from build123d import *

# Parameters (mm, degrees)
F0_R     = 31.75
F0_R_2   = 27.94
F1_DEPTH = 38.1
F2_R     = 31.75
F3_DEPTH = 5.08
F4_R     = 6.35
F5_DEPTH = 61.976


with BuildPart() as f1:
    # F0 (on Front) → F1 (new body)
    with BuildSketch(Plane.XZ):
        Circle(F0_R)
        Circle(F0_R_2, mode=Mode.SUBTRACT)
    extrude(amount=F1_DEPTH)

    # F2 (on Front) → F3 (join)
    with BuildSketch(Plane.XZ):
        with Locations((0.1314867404, -0.3395704844)):
            Circle(F2_R)
    extrude(amount=-F3_DEPTH)

    # F4 (on Top) → F5 (cut, symmetric)
    with BuildSketch(Plane.XY):
        with Locations((0, -20.52645199)):
            Circle(F4_R)
    extrude(amount=F5_DEPTH, both=True, mode=Mode.SUBTRACT)


solid = f1.part
Build history of the part. All positions in model axes, mm. A direction names the side the tool comes from. Round coordinates to 2 decimals unless told otherwise and drop trailing zeros. Write each loop counter-clockwise with the first axis right and the second up, starting at its lowest first coordinate (ties: lowest second). Pieces come first, ordered by that corner, then holes. Notation, with made-up numbers: M -17,-17.75 L -8,-17.75 A22 cw -8,-5.75 Z; hole C 62,-3.75 d3. An arc over 180 degrees is marked long. Answer as a JSON object with one key per item and string values. Group by question number.
(1) Cut at C-C (z = 25.5). Give the cut face in (x, y), and give its area (3 significant figures).
(2) Cut at A-A (x = 0). Give the cut face in (y, z), and give its area (3 significant figures).
(3) Mould opens along Z. For faces 3 (the cylindrical face through (12.89, -18.78, -24.79)), 4 (the cylindrical face through (30.415, 2.504, 9.197)), 5 (the flat face through (-0.1, -38.1, -28.1)) say: pulls with the +Z half, pulls with the -Z half, needs draft (parallel to the pull), parting line crosses it, or undercut.
(4) Flat gauge pins, fed straight in: pin 1 (10 mm diameter, centred on y = -7, z = 1.5, fed in from -X); pin 2 (10 mm diameter, centred on x = 0, y = -20.53, fed in from -Z); pin 3 (8 mm diameter, centred on x = -24, y = -16.5, fed in from +Z); pin 4 (20.5 mm diameter, centred on x = 0, y = -20.53, fed in from -Z). Where does each tip first touch, or does it go through?
(5) Cut at D-D (y = -34). Give the cut face in (x, z).
(6) Drill centre lines: L1, parallel to Y at x = 0, z = -30.2; L2, parallel to X at y = -11, z = 0.5. Where is each one in solid material? Low to high.
(7) Cut at B-B (y = -19). Give the cut face in (x, z).
(8) Which spindle directions (+Z, -Z, +X, -X, +Y, -Y) get a long thin tool onto all of the face, cutting with end or side? Do faces 1 (the cylindrical face through (-6.883, -18.783, -30.995)), 2 (the flat face through (0, 5.08, 0)). Say none if no direction does.
Responses:
{
 "1": {"outline": "M -18.92,-38.1 L -11.42,-38.1 L -11.42,0 L 11.42,0 L 11.42,-38.1 L 18.92,-38.1 L 18.92,0 L 18.58,0 L 18.58,5.08 L -18.32,5.08 L -18.32,0 L -18.92,0 Z", "area": "759 mm2"},
 "2": {"outline": "M -38.1,-31.75 L -26.88,-31.75 L -26.88,-27.94 L -38.1,-27.94 Z; M -38.1,27.94 L -26.88,27.94 L -26.88,31.75 L -38.1,31.75 Z; M -14.18,-31.75 L 0,-31.75 L 0,-32.09 L 5.08,-32.09 L 5.08,31.41 L 0,31.41 L 0,31.75 L -14.18,31.75 L -14.18,27.94 L 0,27.94 L 0,-27.94 L -14.18,-27.94 Z", "area": "516 mm2"},
 "3": {"face 3": "undercut", "face 4": "parting line crosses it", "face 5": "needs draft"},
 "4": {"pin 1": "stops at x = -31.75", "pin 2": "passes through", "pin 3": "stops at z = 24.66", "pin 4": "stops at z = -31.75"},
 "5": {"outline": "C 0,0 d63.5; hole C 0,0 d55.88"},
 "6": {"L1": "y = -38.1 to -26.88, -14.18 to 5.08", "L2": "x = -31.75 to -27.94, 27.94 to 31.75"},
 "7": {"outline": "M -6.16,-31.15 L -6.16,-27.25 A27.94 cw -6.16,27.25 L -6.16,31.15 A31.75 ccw Z; M 6.16,-31.15 A31.75 ccw 6.16,31.15 L 6.16,27.25 A27.94 cw 6.16,-27.25 Z"},
 "8": {"face 1": "-Y", "face 2": "+Z, -Z, +X, -X, +Y"}
}
